```python
from build123d import *

# Parameters (mm, degrees)
EXTRUDE1_DEPTH     = 6.35
CUT_EXTRUDE1_REACH = 327.914
SKETCH2_W          = 25.4
SKETCH2_H          = 6.35
FILLET1_R          = 12.7


with BuildPart() as part:
    # Sketch1 → Extrude1 (new body)
    with BuildSketch(Plane.XY):
        with BuildLine():
            Line((-119.0625, -9.525), (-119.0625, 15.875))
            ThreePointArc((-119.0625, 15.875), (-12.912203714, 33.137302813), (84.185416539, 79.375))
            Line((84.185416539, 79.375), (96.885416539, 79.375))
            Line((96.885416539, 79.375), (96.885416539, 69.85))
            Line((96.885416539, 69.85), (122.285416539, 69.85))
            Line((122.285416539, 69.85), (122.285416539, 79.375))
            Line((122.285416539, 79.375), (238.394583461, 79.375))
            Line((238.394583461, 79.375), (238.394583461, 69.85))
            Line((238.394583461, 69.85), (263.794583461, 69.85))
            Line((263.794583461, 69.85), (263.794583461, 79.375))
            Line((263.794583461, 79.375), (282.844583461, 79.375))
            ThreePointArc((282.844583461, 79.375), (240.685076339, -37.537420224), (238.394583461, -161.797999999))
            Line((238.394583461, -161.797999999), (84.185416539, -161.797999999))
            ThreePointArc((84.185416539, -161.797999999), (-4.377647242, -68.228339866), (-119.0625, -9.525))
        make_face()
    extrude(amount=EXTRUDE1_DEPTH)

    # Sketch2 → Cut-Extrude1 (cut, up to next)
    with BuildSketch(Plane.XY.offset(6.35), mode=Mode.PRIVATE) as cut_extrude1_sk1:
        with Locations((80.9625, 3.175)):
            Rectangle(SKETCH2_W, SKETCH2_H)
    cut_extrude1_tool1 = extrude(cut_extrude1_sk1.sketch, amount=-CUT_EXTRUDE1_REACH, mode=Mode.PRIVATE) & part.part
    # Sketch2 → Cut-Extrude1 (cut, up to next)
    with BuildSketch(Plane.XY.offset(6.35), mode=Mode.PRIVATE) as cut_extrude1_sk2:
        with Locations((-93.6625, 3.175)):
            Rectangle(SKETCH2_W, SKETCH2_H)
    cut_extrude1_tool2 = extrude(cut_extrude1_sk2.sketch, amount=-CUT_EXTRUDE1_REACH, mode=Mode.PRIVATE) & part.part
    add(cut_extrude1_tool1.solids().sort_by_distance((80.9625, 3.175, 6.35))[0], mode=Mode.SUBTRACT)
    add(cut_extrude1_tool2.solids().sort_by_distance((-93.6625, 3.175, 6.35))[0], mode=Mode.SUBTRACT)

    # Fillet1
    # the kernel refuses this fillet: 12.7 mm, written as the material it takes off along each edge
    with BuildSketch(Plane(origin=(-119.0625, -9.525, -23.042479417), x_dir=(0, 1, 0), z_dir=(0, 0, 1))) as fillet1_piece_1:
        with BuildLine():
            CenterArc((9.216991767, -12.7), FILLET1_R, 90, 71.264145378)
            Line((-2.810028359, -8.620687938), (-3.050568761, -8.539101697))
            ThreePointArc((-3.050568761, -8.539101697), (-1.620862846, -4.239985213), (-0.242413755, 0.075839116))
            Line((-0.242413755, 0.075839116), (0, 0.254))
            Line((0, 0.254), (9.216991767, 0.254))
            Line((9.216991767, 0.254), (9.216991767, 0))
        make_face()
    extrude(amount=52.434958835, mode=Mode.SUBTRACT)
    with BuildSketch(Plane(origin=(-119.0625, 15.875, -30.640711511), x_dir=(0, -1, 0), z_dir=(0, 0, 1))) as fillet1_piece_2:
        with BuildLine():
            CenterArc((12.256284605, 12.7), FILLET1_R, 182.936375733, 87.063624267)
            Line((-0.427040748, 12.049417188), (-0.680707255, 12.036405531))
            ThreePointArc((-0.680707255, 12.036405531), (-0.419694109, 6.017401636), (-0.253951201, -0.004978711))
            Line((-0.253951201, -0.004978711), (0, -0.254))
            Line((0, -0.254), (12.256284605, -0.254))
            Line((12.256284605, -0.254), (12.256284605, 0))
        make_face()
    extrude(amount=67.631423023, mode=Mode.SUBTRACT)
    with BuildSketch(Plane(origin=(84.185416539, 79.375, -9.493460645), x_dir=(-0.8358425258463126, -0.5489692814601342, 0), z_dir=(0, 0, 1))) as fillet1_piece_3:
        with BuildLine():
            CenterArc((3.797894625, 12.699847386), FILLET1_R, 236.703669928, 33.015441722)
            Line((-3.17401525, 2.084647308), (-3.313453447, 1.872343306))
            Line((-3.313453447, 1.872343306), (-0.139438197, -0.212304002))
            Line((-0.139438197, -0.212304002), (0.001245211, -0.253996948))
            ThreePointArc((0.001245211, -0.253996948), (1.867817029, -0.249421573), (3.734388846, -0.253996948))
            Line((3.734388846, -0.253996948), (3.735634057, 0))
        make_face()
    extrude(amount=25.33692129, mode=Mode.SUBTRACT)
    with BuildSketch(Plane(origin=(282.844583461, 79.375, -51.250606191), x_dir=(-0.4644541508381782, -0.8855971667576557, 0), z_dir=(0, 0, 1))) as fillet1_piece_4:
        with BuildLine():
            CenterArc((20.841913184, -12.695403149), FILLET1_R, 91.541626127, 107.65176457)
            Line((8.847851573, -16.870626027), (8.607970341, -16.954130484))
            ThreePointArc((8.607970341, -16.954130484), (4.198984106, -8.553284368), (-0.22494168, -0.117971354))
            Line((-0.22494168, -0.117971354), (0.006833414, 0.253908063))
            ThreePointArc((0.006833414, 0.253908063), (10.250121238, 0.116094484), (20.493409062, 0.253908063))
            Line((20.493409062, 0.253908063), (20.500242476, 0))
        make_face()
    extrude(amount=108.851212382, mode=Mode.SUBTRACT)
    with BuildSketch(Plane(origin=(238.394583461, -161.797999999, -36.048448379), x_dir=(-1, 0, 0), z_dir=(0, 0, 1))) as fillet1_piece_5:
        with BuildLine():
            CenterArc((14.419379352, -12.7), FILLET1_R, 90, 96.197539908)
            Line((1.793603229, -14.071049709), (1.541087707, -14.098470704))
            ThreePointArc((1.541087707, -14.098470704), (0.710330378, -7.0592939), (-0.251319787, -0.036801694))
            Line((-0.251319787, -0.036801694), (0, 0.254))
            Line((0, 0.254), (14.419379352, 0.254))
            Line((14.419379352, 0.254), (14.419379352, 0))
        make_face()
    extrude(amount=78.446896758, mode=Mode.SUBTRACT)
    with BuildSketch(Plane(origin=(84.185416539, -161.797999999, -16.813294938), x_dir=(-0.561921339312421, 0.827190672351505, 0), z_dir=(0, 0, 1))) as fillet1_piece_6:
        with BuildLine():
            CenterArc((6.726221855, -12.699521307), FILLET1_R, 90.497468654, 55.313755774)
            Line((-3.779099684, -5.563120298), (-3.989206115, -5.420392277))
            Line((-3.989206115, -5.420392277), (-0.210106431, 0.14272802))
            Line((-0.210106431, 0.14272802), (0.002205319, 0.253990426))
            ThreePointArc((0.002205319, 0.253990426), (3.307977961, 0.239639207), (6.613750604, 0.253990426))
            Line((6.613750604, 0.253990426), (6.615955923, 0))
        make_face()
    extrude(amount=39.976589876, mode=Mode.SUBTRACT)


solid = part.part
```
Build history of the part. All positions in model axes, mm. Round coordinates to 2 decimals unless told otherwise and drop trailing zeros. Order: outer loops, then holes, each group sorted by start corner. A loop starts at its lowest first (then second) coordinate and runs counter-clockwise, first axis right, second up. Notation, with made-up numbers: (5.5, -35.75) - (50.5, -35.75) arc R29 ccw to (50.5, -14.75) - close; hole circle Ø8 at (-16.5, 72). An arc over 180 degrees is marked (long way). Use a Markdown table: item, result.
1) Flat gauge pins, fed straight in: pin 1 Ø3 at (x, y) = (-19, -2) entering from -Z; pin 2 Ø1.9 at (x, z) = (-90, 4.5) entering from +Y; pin 3 Ø1 at (x, z) = (-43, 3) entering from +Y; pin 4 Ø1.9 at (y, z) = (73.5, 1.5) entering from -X. Where does each tip first touch, or does it go through?
Recorded:
| item | result |
|---|---|
| pin 1 | stops at z = 0 |
| pin 2 | stops at y = 17.65 |
| pin 3 | stops at y = 25.18 |
| pin 4 | stops at x = 73.52 |
2) Saw through at A-A on z = 5.25. Give the number of separate pieces and of enclosed holes in the cut face, and give its area (3 significant figures).
Recorded:
| item | result |
|---|---|
| separate pieces | 1 |
| enclosed holes | 2 |
| area | 59,400 mm² |
3) Saw through at B-B on x = 108. Write the cut outline in (y, z), and give its area (3 significant figures).
Recorded:
| item | result |
|---|---|
| outline | (-161.8, 0) - (69.85, 0) - (69.85, 6.35) - (-161.8, 6.35) - close |
| area | 1,470 mm² |
4) Saw through at C-C on y = -54.5. Write the cut outline in (x, z).
Recorded:
| item | result |
|---|---|
| outline | (-23.95, 0) - (237.95, 0) - (237.95, 6.35) - (-23.95, 6.35) - close |
5) Wall check: L1, parallel to Y at x = -102, z = 1.5; L2, parallel to X at y = 0.5, z = 3.5; L3, parallel to Y at x = -88, z = 2.75. Give the ranges that are in metal, low to high.
Recorded:
| item | result |
|---|---|
| L1 | y = -15.31 to 0, 6.35 to 16.59 |
| L2 | x = -119.06 to -106.36, -80.96 to 68.26, 93.66 to 249.74 |
| L3 | y = -20.74 to 0, 6.35 to 17.76 |
